The listing builds one solid part. Answer for the finished solid, in the listing's coordinates (mm). Face numbers are marked on the shaded views. A direction names the side the tool comes from. Give positions to 0.01 mm unless a question says otherwise; leave off trailing zeros. Write each loop counter-clockwise with the first axis right and the second up, starting at its lowest first coordinate (ties: lowest second). Pieces come first, ordered by that corner, then holes. Notation, with made-up numbers: M -28,-32 L 31,-32 A20 cw 31,-4 Z; hole C 25,-13.5 d6. An arc over 180 degrees is marked long. Answer as a JSON object with one key per item and string values.
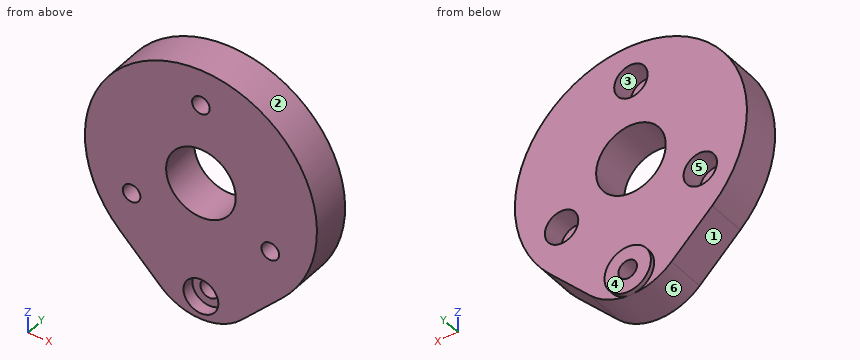
```python
from build123d import *

# Parameters (mm, degrees)
SKETCH_1_R          = 25
SKETCH_1_R_2        = 1.9
SKETCH_1_R_3        = 7.5
EXTRUDE_1_DEPTH     = 8.7
SKETCH_2_R          = 3.6
CUT_EXTRUDE_1_DEPTH = 5
EXTRUDE_START       = -8.7
EXTRUDE_4_DEPTH     = 8.7
SKETCH_14_R         = 2
CUT_EXTRUDE_5_DEPTH = 41.00862407
EXTRUDE_START_2     = 1
SKETCH_15_R         = 5
SKETCH_15_R_2       = 2
EXTRUDE_5_DEPTH     = 1
SKETCH_19_R         = 3.75
CUT_EXTRUDE_7_DEPTH = 2.7


with BuildPart() as part:
    # 草图1 → 凸台-拉伸1 (new body)
    with BuildSketch(Plane(origin=(0, 0, 0), x_dir=(1, 0, 0), z_dir=(0, 1, 0))):
        with Locations(Location((0, 0, 0), (0, 0, 270))):
            Circle(SKETCH_1_R)
        with Locations(Location((14.938938215, 8.625, 0), (0, 0, 270))):
            Circle(SKETCH_1_R_2, mode=Mode.SUBTRACT)
        with Locations(Location((0, -17.25, 0), (0, 0, 270))):
            Circle(SKETCH_1_R_2, mode=Mode.SUBTRACT)
        with Locations(Location((-14.938938215, 8.625, 0), (0, 0, 270))):
            Circle(SKETCH_1_R_2, mode=Mode.SUBTRACT)
        with Locations(Location((0, 0, 0), (0, 0, 270))):
            Circle(SKETCH_1_R_3, mode=Mode.SUBTRACT)
    extrude(amount=EXTRUDE_1_DEPTH)

    # 草图2 → 切除-拉伸1 (cut)
    with BuildSketch(Plane(origin=(0, 8.7, 0), x_dir=(1, 0, 0), z_dir=(0, 1, 0))):
        with Locations(Location((0, -17.25, 0), (0, 0, 270))):
            Circle(SKETCH_2_R)
        with Locations(Location((-14.938938215, 8.625, 0), (0, 0, 270))):
            Circle(SKETCH_2_R)
        with Locations(Location((14.938938215, 8.625, 0), (0, 0, 270))):
            Circle(SKETCH_2_R)
    extrude(amount=-CUT_EXTRUDE_1_DEPTH, mode=Mode.SUBTRACT)

    # 草图13 → 凸台-拉伸4 (add)
    with BuildSketch(Plane(origin=(0, 8.7, 0), x_dir=(1, 0, 0), z_dir=(0, 1, 0)).offset(EXTRUDE_START)):
        with BuildLine():
            Line((-8.748177653, 26.428571429), (-17.496355306, 17.857142857))
            ThreePointArc((-17.496355306, 17.857142857), (0, 25), (17.496355306, 17.857142857))
            Line((17.496355306, 17.857142857), (8.748177653, 26.428571429))
            ThreePointArc((8.748177653, 26.428571429), (0, 30), (-8.748177653, 26.428571429))
        make_face()
    extrude(amount=EXTRUDE_4_DEPTH)

    # 草图14 → 切除-拉伸5 (cut, through all)
    with BuildSketch(Plane(origin=(0, 8.7, 0), x_dir=(1, 0, 0), z_dir=(0, 1, 0))):
        with Locations(Location((0, 25, 0), (0, 0, 270))):
            Circle(SKETCH_14_R)
    extrude(amount=-CUT_EXTRUDE_5_DEPTH, mode=Mode.SUBTRACT)

    # 草图15 → 凸台-拉伸5 (add)
    with BuildSketch(Plane(origin=(0, 8.7, 0), x_dir=(1, 0, 0), z_dir=(0, 1, 0)).offset(EXTRUDE_START_2)):
        with Locations(Location((0, 25, 0), (0, 0, 89.99953218))):
            Circle(SKETCH_15_R)
        with Locations(Location((0, 25, 0), (0, 0, 270))):
            Circle(SKETCH_15_R_2, mode=Mode.SUBTRACT)
    extrude(amount=-EXTRUDE_5_DEPTH)

    # 草图19 → 切除-拉伸7 (cut)
    with BuildSketch(Plane.XZ):
        with Locations(Location((0, -25, 0), (0, 0, 270))):
            Circle(SKETCH_19_R)
    extrude(amount=-CUT_EXTRUDE_7_DEPTH, mode=Mode.SUBTRACT)


solid = part.part
```
1. A cutting plane is placed at A-A, the plane z = 0. Give the vertices of the cut face in (x, y), plus the area to 4 significant figures.
Verdict:
{"outline": "M -25,0 L -7.5,0 L -7.5,8.7 L -25,8.7 Z; M 7.5,0 L 25,0 L 25,8.7 L 7.5,8.7 Z", "area": "304.5 mm2"}
2. Consider line 1 along Z through (x, y) = (1.5, 2.5); line 2 along Y through (x, z) = (-20, -1.5); line 3 along Z through (x, y) = (15, 5). Determine where each line is inside the solid, lowest interval first.
Verdict:
{"line 1": "z = -29.91 to -28.44, -21.56 to -7.35, 7.35 to 16.08, 18.42 to 24.95", "line 2": "y = 0 to 8.7", "line 3": "z = -20.3 to -12.22, -5.03 to 20"}
3. Flat-ended cylindrical pins translate along their axes: pin 1 (4 mm diameter, centred on x = -8, y = 3.5, fed in from +Z); pin 2 (2 mm diameter, centred on x = 0, z = -26.5, fed in from -Y); pin 3 (25 mm diameter, centred on x = 2.5, z = -6, fed in from +Y); pin 4 (3 mm diameter, centred on x = 0, z = -25, fed in from -Y). Find the tip coordinate at first contact, or state that the pin passes through.
Verdict:
{"pin 1": "stops at z = 24.27", "pin 2": "stops at y = 2.7", "pin 3": "stops at y = 8.7", "pin 4": "passes through"}
4. A cutting plane is placed at C-C, the plane y = 1.25. Give the vertices of the cut face in (x, z) (3 decimals).
Verdict:
{"outline": "M -17.496,-17.857 L -8.748,-26.429 A12.5 ccw 8.748,-26.429 L 17.496,-17.857 A25 ccw long Z; hole C -14.939,-8.625 d3.8; hole C 0,0 d15; hole C 0,-25 d7.5; hole C 0,17.25 d3.8; hole C 14.939,-8.625 d3.8"}
5. A cutting plane is placed at B-B, the plane x = -6. Give the vertices of the cut face in (y, z).
Verdict:
{"outline": "M 0,-28.47 L 8.7,-28.47 L 8.7,-4.5 L 0,-4.5 Z; M 0,4.5 L 8.7,4.5 L 8.7,24.27 L 0,24.27 Z"}
6. The mould has two halves that part along X. Classify the marked faces 1, 2, 3 and 4: released by +X, released by -X, zero draft, split by the parting line, or undercut.
Verdict:
{"face 1": "released by -X", "face 2": "split by the parting line", "face 3": "undercut", "face 4": "zero draft"}
7. A cutting plane is placed at D-D, the plane z = 18.5. Give the vertices of the cut face in (x, y).
Verdict:
{"outline": "M -16.82,0 L -1.43,0 L -1.43,3.7 L -3.38,3.7 L -3.38,8.7 L -16.82,8.7 Z; M 1.43,0 L 16.82,0 L 16.82,8.7 L 3.38,8.7 L 3.38,3.7 L 1.43,3.7 Z"}
8. For the marked faces 5 and 6, determine the directions among +Z, -Z, +X, -X, +Y, -Y from which every point of the face is accessible in a straight line to the end or side of a thin tool.
Verdict:
{"face 5": "+Y", "face 6": "-Z, +Y, -Y"}
